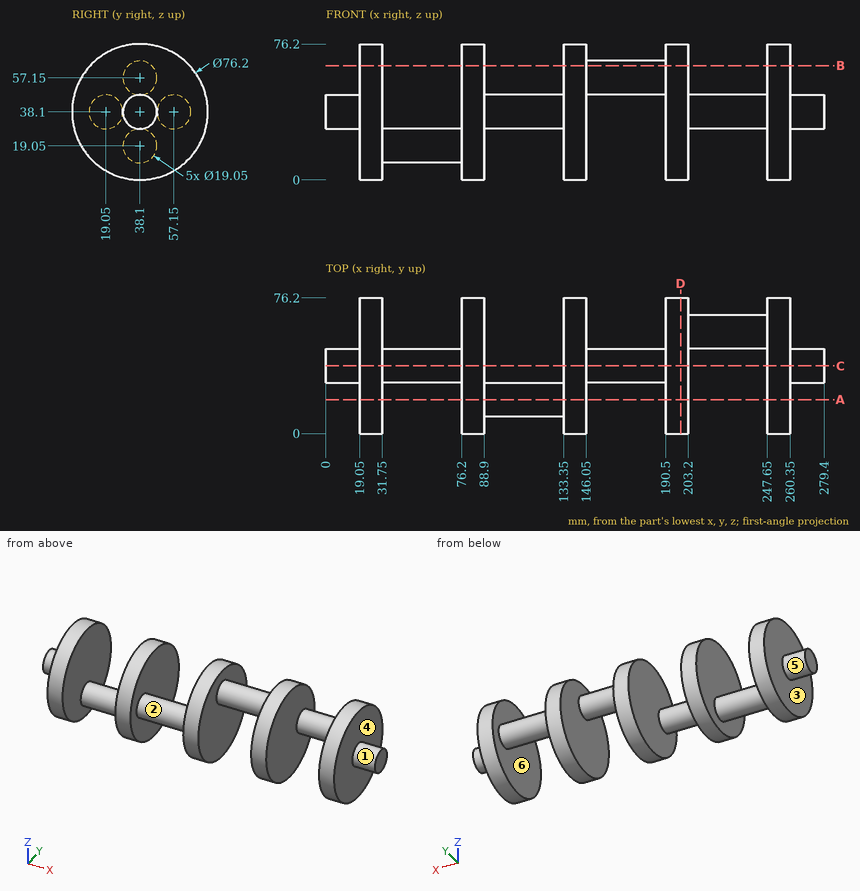
Source: three-view drawing plus pictorial views. Frame: mm from the lowest corner of the part. A direction names the side the tool comes from. Round coordinates to 2 decimals unless told otherwise and drop trailing zeros. Loops run counter-clockwise (first coordinate to the right, second up) from the corner with the lowest first, then second, coordinate; pieces in that order, holes last.
Item 1: Line query: L1, parallel to X at y = 57, z = 13.5; L2, parallel to X at y = 11, z = 39; L3, parallel to X at y = 44, z = 13. Output: solid intervals per line, ascending.
Checked values:
L1: x = 19.05 to 31.75, 76.2 to 88.9, 133.35 to 146.05, 190.5 to 203.2, 247.65 to 260.35
L2: x = 19.05 to 31.75, 76.2 to 146.05, 190.5 to 203.2, 247.65 to 260.35
L3: x = 19.05 to 88.9, 133.35 to 146.05, 190.5 to 203.2, 247.65 to 260.35
Item 2: Section A-A, the plane y = 19.05. Output: boundary loops of the cut face in (x, z) (3 decimals), plus the area to 3 significant figures.
Checked values:
outline: (19.05, 5.104) - (31.75, 5.104) - (31.75, 71.096) - (19.05, 71.096) - close; (76.2, 5.104) - (88.9, 5.104) - (88.9, 28.575) - (133.35, 28.575) - (133.35, 5.104) - (146.05, 5.104) - (146.05, 71.096) - (133.35, 71.096) - (133.35, 47.625) - (88.9, 47.625) - (88.9, 71.096) - (76.2, 71.096) - close; (190.5, 5.104) - (203.2, 5.104) - (203.2, 71.096) - (190.5, 71.096) - close; (247.65, 5.104) - (260.35, 5.104) - (260.35, 71.096) - (247.65, 71.096) - close
area: 5,040 mm2
Item 3: Mould query, pull axis X, two halves, no side actions, for the marked faces 4, 5 and 6. Classes: released by +X, released by -X, zero draft, split by the parting line, or undercut.
Checked values:
face 4: released by +X
face 5: zero draft
face 6: undercut
Item 4: Section B-B, the plane z = 64. Output: boundary loops of the cut face in (x, y), plus the area to 3 significant figures.
Checked values:
outline: (19.05, 10.16) - (31.75, 10.16) - (31.75, 66.04) - (19.05, 66.04) - close; (76.2, 10.16) - (88.9, 10.16) - (88.9, 66.04) - (76.2, 66.04) - close; (133.35, 10.16) - (146.05, 10.16) - (146.05, 31.48) - (190.5, 31.48) - (190.5, 10.16) - (203.2, 10.16) - (203.2, 66.04) - (190.5, 66.04) - (190.5, 44.72) - (146.05, 44.72) - (146.05, 66.04) - (133.35, 66.04) - close; (247.65, 10.16) - (260.35, 10.16) - (260.35, 66.04) - (247.65, 66.04) - close
area: 4,140 mm2
Item 5: Section D-D, the plane x = 199. Output: boundary loops of the cut face in (y, z).
Checked values:
outline: circle Ø76.2 at (38.1, 38.1)
Item 6: Section C-C, the plane y = 38.1. State how many separate pieces and enclosed holes the cut face has, plus the area to 3 significant figures.
Checked values:
separate pieces: 3
enclosed holes: 0
area: 7,260 mm2
Item 7: Reachability of the marked faces 1, 2 and 3 from +Z, -Z, +X, -X, +Y, -Y: full face, straight path, thin tool, end or side. Return the list, or none.
Checked values:
face 1: +X
face 2: none
face 3: -X
Item 8: Contact query for flat-ended pins moving along their axis: P1, Ø1, axis at y = 28.5, z = 62, coming from the -X side; P2, Ø1.5, axis at x = 208, y = 68, coming from the +Z side; P3, Ø6, axis at y = 49, z = 21.5, coming from the +X side; P4, Ø8, axis at x = 103.5, z = 48.5, coming from the -Y side. Output: stop coordinate, or through.
Checked values:
P1: stops at x = 19.05
P2: passes through
P3: stops at x = 260.35
P4: stops at y = 12
